from build123d import *

# Parameters (mm, degrees)
BOSS_EXTRUDE1_DEPTH = 200
CHAMFER1_SIZE       = 1
LPATTERN1_COUNT     = 2
LPATTERN1_PITCH     = 85
LPATTERN2_COUNT     = 2
LPATTERN2_PITCH     = 170


with BuildPart() as part:
    # Sketch1 → Boss-Extrude1 (new body)
    with BuildSketch(Plane(origin=(-15, 0, 0), x_dir=(0, 0, -1), z_dir=(1, 0, 0))):
        with BuildLine():
            Line((-7.4, -7.5), (-7.4, -10))
            Line((-7.4, -10), (0, -10))
            Line((0, -10), (0, 10))
            Line((0, 10), (-7.4, 10))
            Line((-7.4, 10), (-7.4, 7.5))
            Line((-7.4, 7.5), (-6.191570324, 7.5))
            ThreePointArc((-6.191570324, 7.5), (-4.75, 8.375), (-3.308429676, 7.5))
            Line((-3.308429676, 7.5), (-1.4, 7.5))
            Line((-1.4, 7.5), (-1.4, -7.5))
            Line((-1.4, -7.5), (-3.308429676, -7.5))
            ThreePointArc((-3.308429676, -7.5), (-4.75, -8.375), (-6.191570324, -7.5))
            Line((-6.191570324, -7.5), (-7.4, -7.5))
        make_face()
    extrude(amount=BOSS_EXTRUDE1_DEPTH)

    # Chamfer1
    chamfer1_edges = [part.edges().sort_by_distance(p)[0] for p in [
        (85, 10, 0),
        (85, -10, 0),
    ]]
    chamfer(chamfer1_edges, length=CHAMFER1_SIZE)

    # Sketch2 → Cut-Revolve1 (revolve, cut)
    with BuildSketch(Plane(origin=(0, 0, 0), x_dir=(0, 0, -1), z_dir=(1, 0, 0))):
        Polygon((-1.4, 3.05), (0, 1.65), (0, 0), (-1.4, 0), align=None)
    cut_revolve1 = revolve(axis=Axis((0, 0, 0), (0, 0, 1)), mode=Mode.SUBTRACT)

    # LPattern1: Cut-Revolve1 ×2
    with Locations(*[(i * LPATTERN1_PITCH, 0, 0) for i in range(1, LPATTERN1_COUNT)]):
        add(cut_revolve1, mode=Mode.SUBTRACT)

    # LPattern2: Cut-Revolve1 ×2
    with Locations(*[(i * LPATTERN2_PITCH, 0, 0) for i in range(1, LPATTERN2_COUNT)]):
        add(cut_revolve1, mode=Mode.SUBTRACT)


solid = part.part
Geometry check sheet. Reference: the model listing, model coordinates, mm. A direction names the side the tool comes from. Coordinates: 2 decimals unless noted, no trailing zeros. Write each loop counter-clockwise with the first axis right and the second up, starting at its lowest first coordinate (ties: lowest second). Pieces come first, ordered by that corner, then holes. Notation, with made-up numbers: (-39.75, -6) -> (-8.75, -6) arc R17 cw to (-8.75, 11) -> close; hole circle Ø10 at (4.25, -16). An arc over 180 degrees is marked (long way). One line per question, with ' | ' between items.
1. Cross-section at B-B on x = 170. Record the cut outline in (y, z) (3 decimals), and give its area (3 significant figures).
Answers:
outline: (-10, 1) -> (-9, 0) -> (-1.65, 0) -> (-3.05, 1.4) -> (-7.5, 1.4) -> (-7.5, 3.308) arc R1.625 cw to (-7.5, 6.192) -> (-7.5, 7.4) -> (-10, 7.4) -> close; (1.65, 0) -> (9, 0) -> (10, 1) -> (10, 7.4) -> (7.5, 7.4) -> (7.5, 6.192) arc R1.625 cw to (7.5, 3.308) -> (7.5, 1.4) -> (3.05, 1.4) -> close | area: 46.8 mm²
2. Depth check by flat-ended pin: pin 1 Ø4 at (x, y) = (43.5, -5) entering from +Z; pin 2 Ø3 at (y, z) = (-2, 2) entering from -X. Enter the tip coordinate at first touch or a pass-through.
Answers:
pin 1: stops at z = 1.4 | pin 2: stops at x = -15
3. Set-up check for faces 1 (the flat face through (84, -2, 0)), 2 (the flat face through (83.6, 3.4, 1.4)): record each of +Z, -Z, +X, -X, +Y, -Y from which the full face is reachable in a straight line by a thin tool's end or side.
Answers:
face 1: -Z, +X, -X, +Y, -Y | face 2: +Z, +X, -X
4. Cross-section at C-C on z = 4.5. Record the cut outline in (x, y).
Answers:
outline: (-15, -10) -> (185, -10) -> (185, -8.36) -> (-15, -8.36) -> close; (-15, 8.36) -> (185, 8.36) -> (185, 10) -> (-15, 10) -> close
5. Thickness scan on probe 1 along Y at (x, z) = (116, 6.25); probe 2 along Z at (x, y) = (170, -6.5); probe 3 along Y at (x, z) = (62, 4.25). Record the ranges inside material, lowest first. Write a range as from..to.
Answers:
probe 1: y = -10..-7.5, 7.5..10 | probe 2: z = 0..1.4 | probe 3: y = -10..-8.3, 8.3..10
6. Cross-section at A-A on y = 0. Record the cut outline in (x, z), and give its area (3 significant figures).
Answers:
outline: (-15, 0) -> (-1.65, 0) -> (-3.05, 1.4) -> (-15, 1.4) -> close; (1.65, 0) -> (83.35, 0) -> (81.95, 1.4) -> (3.05, 1.4) -> close; (86.65, 0) -> (168.35, 0) -> (166.95, 1.4) -> (88.05, 1.4) -> close; (171.65, 0) -> (185, 0) -> (185, 1.4) -> (173.05, 1.4) -> close | area: 260 mm²
7. Cross-section at D-D on x = 25. Record the cut outline in (y, z) (3 decimals), and give its area (3 significant figures).
Answers:
outline: (-10, 1) -> (-9, 0) -> (9, 0) -> (10, 1) -> (10, 7.4) -> (7.5, 7.4) -> (7.5, 6.192) arc R1.625 cw to (7.5, 3.308) -> (7.5, 1.4) -> (-7.5, 1.4) -> (-7.5, 3.308) arc R1.625 cw to (-7.5, 6.192) -> (-7.5, 7.4) -> (-10, 7.4) -> close | area: 53.4 mm²
